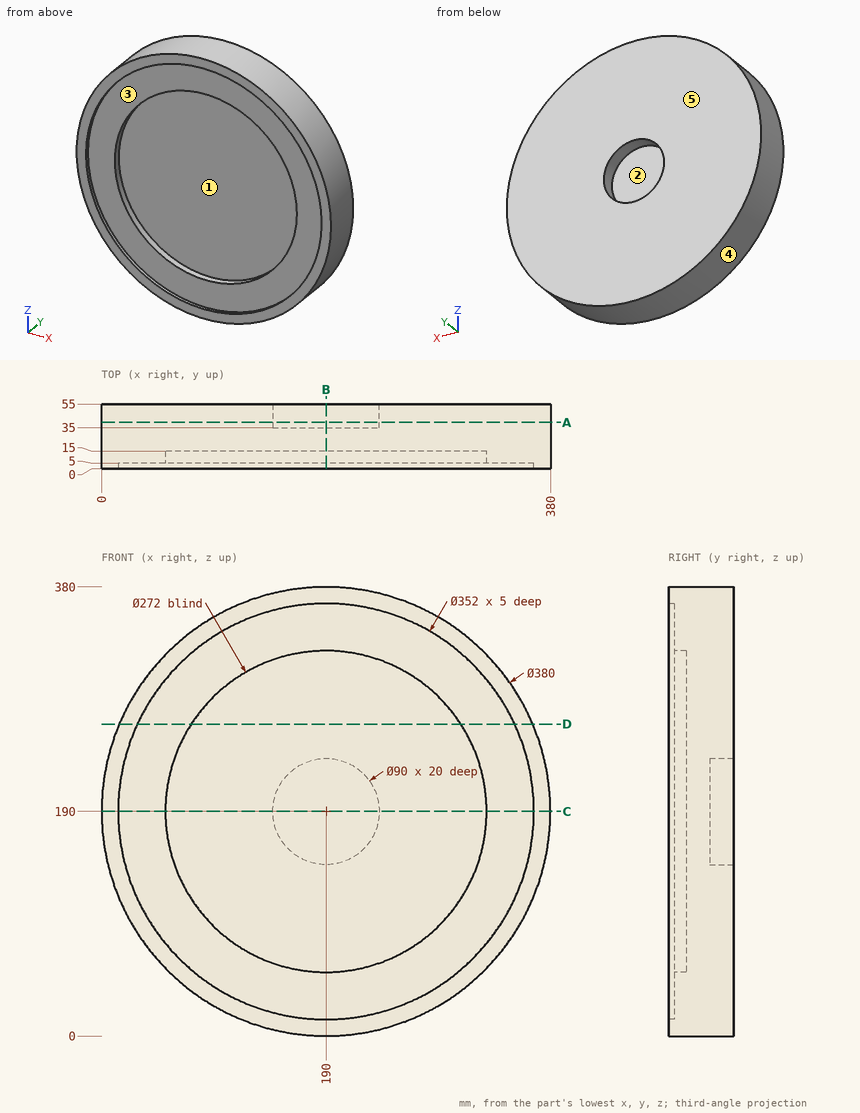
The drawing under review shows one solid part. Ordinate dimensions are in mm from its lowest x, y, z. A direction names the side the tool comes from. Round coordinates to 2 decimals unless told otherwise and drop trailing zeros. Loops run counter-clockwise (first coordinate to the right, second up) from the corner with the lowest first, then second, coordinate; pieces in that order, holes last. Notation, with made-up numbers: (-31, 23) - (-18, 23) arc R33 cw to (-18, 51) - close; hole circle Ø3 at (36.5, 15). An arc over 180 degrees is marked (long way). Put each result on its own line as item: value. Start each with the question number.
1. For the marked faces 1 and 2, list the 3-axis set-ups (+Z, -Z, +X, -X, +Y, -Y) from which the entire face can be reached by the end or side of a thin tool; tool diameter is ignored.
2. Insertion check: P1, Ø4, axis at y = 20.5, z = 46, coming from the -X side; P2, Ø4, axis at x = 70, y = 23.5, coming from the -Z side; P3, Ø1, axis at y = 30, z = 213.5, coming from the +X side. Each pin has a flat end and moves straight along its axis. Give the tip position at first contact, or say it passes through.
3. For probe 1 along Z at (x, y) = (190, 39.5); probe 2 along Z at (x, y) = (190, 7); probe 3 along X at (y, z) = (47, 230), list the stretches that pass through material, from the lowest coordinate up. Write a range as [from, to].
4. Consider section A-A on y = 39.5. State the section outline as (x, z) points, plus the area to 3 significant figures.
5. Consider section B-B on x = 190. State the section outline as (y, z) points.
6. Consider section D-D on z = 264. State the section outline as (x, y) points, plus the area to 3 significant figures.
7. Consider section C-C on z = 190. State the section outline as (x, y) points, plus the area to 3 significant figures.
8. Mouldability with a two-part tool opening along Z and no side actions: class the marked faces 3, 4 and 5 as +Z half, -Z half, draft (parallel to the pull), parting line (faces both ways), or undercut.
Result sheet:
1. face 1: -Y
1. face 2: +Y
2. P1: x = 63.76
2. P2: z = 41.08
2. P3: x = 378.6
3. probe 1: [0, 145], [235, 380]
3. probe 2: [0, 54], [326, 380]
3. probe 3: [4.26, 169.38], [210.62, 375.74]
4. outline: circle Ø380 at (190, 190); hole circle Ø90 at (190, 190)
4. area: 107,000 mm^2
5. outline: (0, 0) - (55, 0) - (55, 145) - (35, 145) - (35, 235) - (55, 235) - (55, 380) - (0, 380) - (0, 366) - (5, 366) - (5, 326) - (15, 326) - (15, 54) - (5, 54) - (5, 14) - (0, 14) - close
6. outline: (15, 0) - (30.31, 0) - (30.31, 5) - (75.89, 5) - (75.89, 15) - (304.11, 15) - (304.11, 5) - (349.69, 5) - (349.69, 0) - (365, 0) - (365, 55) - (15, 55) - close
6. area: 15,400 mm^2
7. outline: (0, 0) - (14, 0) - (14, 5) - (54, 5) - (54, 15) - (326, 15) - (326, 5) - (366, 5) - (366, 0) - (380, 0) - (380, 55) - (235, 55) - (235, 35) - (145, 35) - (145, 55) - (0, 55) - close
7. area: 14,600 mm^2
8. face 3: undercut
8. face 4: parting line
8. face 5: draft
